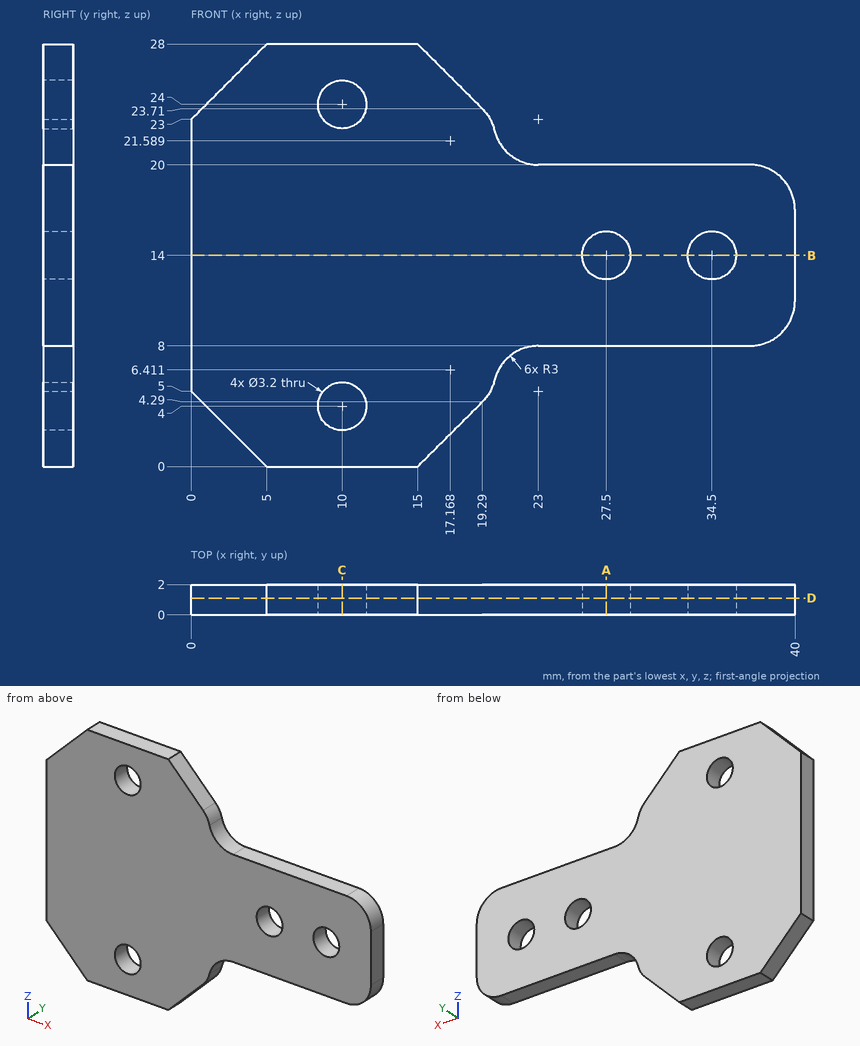
Geometry: see drawing. Coordinates: mm, zero at the bounding-box minimum. Round coordinates to 2 decimals unless told otherwise and drop trailing zeros. Order: outer loops, then holes, each group sorted by start corner. A loop starts at its lowest first (then second) coordinate and runs counter-clockwise, first axis right, second up. Notation, with made-up numbers: (-25, 72) -> (-8, 72) arc R34 cw to (-8, 102) -> close; hole circle Ø7 at (-26.5, 37). An arc over 180 degrees is marked (long way). Answer as CSV lines item,"result".
Item 1: Line query: L1, parallel to X at y = 1.15, z = 14; L2, parallel to Z at x = 25, y = 1.4; L3, parallel to X at y = 0.55, z = 15. Output: solid intervals per line, ascending.
A:
L1,"0 to 25.9, 29.1 to 32.9, 36.1 to 40"
L2,"8 to 20"
L3,"0 to 26.25, 28.75 to 33.25, 35.75 to 40"
Item 2: Section B-B, the plane z = 14. Return loops of the section in (x, y).
A:
outline,"(0, 0) -> (25.9, 0) -> (25.9, 2) -> (0, 2) -> close; (29.1, 0) -> (32.9, 0) -> (32.9, 2) -> (29.1, 2) -> close; (36.1, 0) -> (40, 0) -> (40, 2) -> (36.1, 2) -> close"
Item 3: Section A-A, the plane x = 27.5. Return loops of the section in (y, z).
A:
outline,"(0, 8) -> (2, 8) -> (2, 12.4) -> (0, 12.4) -> close; (0, 15.6) -> (2, 15.6) -> (2, 20) -> (0, 20) -> close"
Item 4: Section D-D, the plane y = 1.1. Return loops of the section in (x, z) (1 decimal).
A:
outline,"(0, 5) -> (5, 0) -> (15, 0) -> (19.3, 4.3) arc R3 ccw to (20.1, 5.7) arc R3 cw to (23, 8) -> (37, 8) arc R3 ccw to (40, 11) -> (40, 17) arc R3 ccw to (37, 20) -> (23, 20) arc R3 cw to (20.1, 22.3) arc R3 ccw to (19.3, 23.7) -> (15, 28) -> (5, 28) -> (0, 23) -> close; hole circle Ø3.2 at (10, 4); hole circle Ø3.2 at (10, 24); hole circle Ø3.2 at (27.5, 14); hole circle Ø3.2 at (34.5, 14)"
Item 5: Section C-C, the plane x = 10. Return loops of the section in (y, z), plus the area to 3 significant figures.
A:
outline,"(0, 0) -> (2, 0) -> (2, 2.4) -> (0, 2.4) -> close; (0, 5.6) -> (2, 5.6) -> (2, 22.4) -> (0, 22.4) -> close; (0, 25.6) -> (2, 25.6) -> (2, 28) -> (0, 28) -> close"
area,"43.2 mm²"
Item 6: Pin query (flat end, axial travel): pin 1 Ø1 at (x, y) = (18, 0.5) entering from -Z. Return the tip coordinate at first contact, or that it passes through.
A:
pin 1,"z = 2.5"
